```python
from build123d import *
from build123d import SkipClean  # not in build123d's __all__

# Parameters (mm, degrees)
F0_W     = 90
F0_H     = 90
F0_W_2   = 86
F0_H_2   = 86
F1_DEPTH = 97
F2_W     = 86
F2_H     = 86
F2_R     = 4
F3_DEPTH = 2
F7_R     = 2.5
F8_DEPTH = 76.2


with BuildPart() as f1:
    # F0 (on Top) → F1 (new body)
    with BuildSketch(Plane.XY):
        Rectangle(F0_W, F0_H)
        Rectangle(F0_W_2, F0_H_2, mode=Mode.SUBTRACT)
    extrude(amount=F1_DEPTH)

    # F2 (on face) → F3 (join)
    with BuildSketch(Plane.XY.offset(97)):
        Rectangle(F2_W, F2_H)
        Circle(F2_R, mode=Mode.SUBTRACT)
    extrude(amount=-F3_DEPTH)

    # F4 (on Front) → F6 (revolve)
    with BuildSketch(Plane.XZ):
        Polygon((-2.5, 97), (-4, 97), (-4, 95), (-4, 93.5), (-4.4, 93.5), (-4, 90), (-4.4, 90), (-4, 86.5), (-2.5, 86.5), align=None)
    revolve(axis=Axis((0, 0, 51.8437661231), (0, 0, 1)))

    # F7 (on Front) → F8 (cut)
    with BuildSketch(Plane.XZ):
        with Locations((6.35, 43.18)):
            Circle(F7_R)
    extrude(amount=F8_DEPTH, mode=Mode.SUBTRACT)

    # F11 (on offset) → F12 (revolve)
    with BuildSketch(Plane.YZ.offset(6.35)):
        Polygon((-39.5560968816, 47.18), (-43.0560968816, 47.18), (-43.0560968816, 45.68), (-32.5560968816, 45.68), (-32.5560968816, 47.18), (-36.0560968816, 47.18), align=None)
        Polygon((-39.5560968816, 47.58), (-39.5560968816, 47.18), (-36.0560968816, 47.18), align=None)
        Polygon((-36.0560968816, 47.58), (-36.0560968816, 47.18), (-32.5560968816, 47.18), align=None)
    with SkipClean():  # cleaning this boolean's faces spoils the solid; the shape is the same uncleaned
        revolve(axis=Axis((6.35, -16.5081392042, 43.18), (0, 1, 0)))


solid = f1.part
```
Geometry: final body of the model. Coordinates: model frame, mm. A direction names the side the tool comes from. Coordinates: 2 decimals unless noted, no trailing zeros. Order: outer loops, then holes, each group sorted by start corner. A loop starts at its lowest first (then second) coordinate and runs counter-clockwise, first axis right, second up. Notation, with made-up numbers: M 19.5,74.5 L 75.5,74.5 A13 ccw 75.5,99.5 Z; hole C 17.5,-22 d2. An arc over 180 degrees is marked long. Answer in a Markdown table with one row per item. Add a question column.
Q1. Section query A-A on y = 0. Return the cut outline in (x, z).
Q2. Mould query, pull axis Y, two halves, no side actions, for faces 1 (the flat face through (9, 1, 95)), 2 (the flat face through (-1, 45, 48)), 3 (the flat face through (8, -32.556, 41)), 4 (the flat face through (45, -1, 48)). Classes: released by +Y, released by -Y, zero draft, split by the parting line, or undercut.
Q3. Line query: L1, parallel to Y at x = 1, z = 77.5; L2, parallel to X at y = -41.5, z = 43.18. Output: solid intervals per line, ascending.
Q4. Section query C-C on z = 66. Return the cut outline in (x, y).
Q5. Section query D-D on z = 43.18. Return the cut outline in (x, y).
Q6. Contact query for flat-ended pins moving along their axis: P1, Ø6, axis at x = -34, y = -30.5, coming from the -Z side; P2, Ø6.5, axis at x = -0.5, y = 1, coming from the -Z side. Output: stop coordinate, or through.
Q7. Reachability of faces 5 (the cylindrical face through (8.32, -38.69, 41.64)), 6 (the flat face through (-43, -1, 47)), 7 (the conical face through (-3.96, -1.25, 91.34)) from +Z, -Z, +X, -X, +Y, -Y: full face, straight path, thin tool, end or side. Return the list, or none.
Completed:
| question | item | result |
|---|---|---|
| 1 | outline | M -45,0 L -43,0 L -43,95 L -4,95 L -4,93.5 L -4.4,93.5 L -4,90 L -4.4,90 L -4,86.5 L -2.5,86.5 L -2.5,97 L -45,97 Z; M 2.5,86.5 L 4,86.5 L 4.4,90 L 4,90 L 4.4,93.5 L 4,93.5 L 4,95 L 43,95 L 43,0 L 45,0 L 45,97 L 2.5,97 Z |
| 2 | face 1 | undercut |
| 2 | face 2 | released by +Y |
| 2 | face 3 | undercut |
| 2 | face 4 | zero draft |
| 3 | L1 | y = -45 to -43, 43 to 45 |
| 3 | L2 | x = -45 to -43, 2.35 to 3.85, 8.85 to 10.35, 43 to 45 |
| 4 | outline | M -45,-45 L 45,-45 L 45,45 L -45,45 Z; hole M -43,-43 L 43,-43 L 43,43 L -43,43 Z |
| 5 | outline | M -45,-45 L 3.85,-45 L 3.85,-32.56 L 2.35,-32.56 L 1.95,-36.06 L 2.35,-36.06 L 1.95,-39.56 L 2.35,-39.56 L 2.35,-43 L -43,-43 L -43,43 L 43,43 L 43,-43 L 10.35,-43 L 10.35,-39.56 L 10.75,-39.56 L 10.35,-36.06 L 10.75,-36.06 L 10.35,-32.56 L 8.85,-32.56 L 8.85,-45 L 45,-45 L 45,45 L -45,45 Z |
| 6 | P1 | stops at z = 95 |
| 6 | P2 | stops at z = 86.5 |
| 7 | face 5 | -Y |
| 7 | face 6 | -Z |
| 7 | face 7 | none |
